```python
from build123d import *

# Parameters (mm, degrees)
SKETCH_R           = 9
PAD_DEPTH          = 6
POCKET_DEPTH       = 6
POLARPATTERN_COUNT = 16
SKETCH002_R        = 4
PAD001_DEPTH       = 6
SKETCH004_R        = 2
POCKET002_DEPTH    = 5
POCKET003_DEPTH    = 0.5
SKETCH003_R        = 1.25
POCKET004_DEPTH    = 15


with BuildPart() as part:
    # Sketch → Pad (new body)
    with BuildSketch(Plane.XY):
        Circle(SKETCH_R)
    extrude(amount=-PAD_DEPTH)

    # Sketch001 (on Face6 of Pad) → Pocket (cut)
    with BuildSketch(Plane.XY):
        Polygon((-0.5, 6.5), (0.5, 6.5), (0.75, 7.5), (1.25, 9), (-1.25, 9), (-0.75, 7.5), align=None)
    pocket = extrude(amount=-POCKET_DEPTH, mode=Mode.SUBTRACT)

    # PolarPattern: Pocket ×16 about axis
    polarpattern_axis = Axis((0, 0, 0), (0, 0, 1))
    for i in range(1, POLARPATTERN_COUNT):
        add(pocket.rotate(polarpattern_axis, i * 360 / POLARPATTERN_COUNT), mode=Mode.SUBTRACT)

    # Sketch002 → Pad001 (join)
    with BuildSketch(Plane.XY):
        Circle(SKETCH002_R)
    extrude(amount=PAD001_DEPTH)

    # Sketch004 → Pocket002 (cut)
    with BuildSketch(Plane.XZ):
        with Locations((0, 2.75)):
            Circle(SKETCH004_R)
    extrude(amount=POCKET002_DEPTH, mode=Mode.SUBTRACT)

    # Sketch004 → Pocket003 (cut)
    with BuildSketch(Plane.XZ):
        with Locations((0, 2.75)):
            Circle(SKETCH004_R)
    extrude(amount=-POCKET003_DEPTH, mode=Mode.SUBTRACT)

    # Sketch003 (on Face100 of Pad001) → Pocket004 (cut)
    with BuildSketch(Plane.XY.offset(6)):
        Circle(SKETCH003_R)
    extrude(amount=-POCKET004_DEPTH, mode=Mode.SUBTRACT)


solid = part.part
```
Read the model definition and answer for the solid it produces. Units are mm, in the model's axes. A direction names the side the tool comes from. Round coordinates to 2 decimals unless told otherwise and drop trailing zeros. Write each loop counter-clockwise with the first axis right and the second up, starting at its lowest first coordinate (ties: lowest second). Pieces come first, ordered by that corner, then holes. Notation, with made-up numbers: (16.5, 49.5) -> (24.5, 49.5) arc R16 ccw to (24.5, 59.5) -> close; hole circle Ø8 at (-12.5, 37). An arc over 180 degrees is marked (long way). Answer in a Markdown table with one row per item. Add a question column.
1) Which of the six approach directions +Z, -Z, +X, -X, +Y, -Y give full straight-line access (tool end or side, diameter ignored) to faces 4 (the face through (6.993, -0.623, -2.958)), 5 (the face through (6.7, 2.1, -3)), 6 (the face through (-6.993, 0.623, -2.958))?
2) Find section C-C, the plane z = 5. Determine the outline of the cut face in (x, y), and give its area (3 significant figures).
3) Determine the mould class of faces 1 (the face through (0.983, 8.198, -2.958)), 2 (the face through (5.1, -6.49, -2.96)), 3 (the face through (-6.23, -3.26, -2.96)) for opening direction X: pulls with the +X half, pulls with the -X half, needs draft (parallel to the pull), parting line crosses it, or undercut.
4) Consider line 1 (Y direction, x = 0, z = -0.25); line 2 (X direction, y = 4.5, z = -3.25); line 3 (X direction, y = 6.25, z = -2). Determine where each line is inside the solid, lowest interval first.
5) Find section B-B, the plane y = 0. Determine the outline of the cut face in (x, z), and give its area (3 significant figures).
6) Find section A-A, the plane x = 0. Determine the outline of the cut face in (y, z), and give its area (3 significant figures).
7) Find section D-D, the plane z = 2.75. Determine the outline of the cut face in (x, y), and give its area (3 significant figures).
8) Given P1, Ø1.5, axis at x = 2.5, z = -3, coming from the -Y side; P2, Ø8, axis at x = -6.5, y = -0.5, coming from the +Z side; P3, Ø5, axis at x = 0, z = 2.75, coming from the +Y side; P4, Ø0.5, axis at x = 0, z = -1.5, coming from the +Y side, each flat-ended and moving along its own axis, determine where each tip first touches the part or whether it passes through.
Findings below:
| question | item | result |
|---|---|---|
| 1 | face 4 | +Z, -Z, +X |
| 1 | face 5 | +Z, -Z |
| 1 | face 6 | +Z, -Z, -X |
| 2 | outline | circle Ø8 at (0, 0); hole circle Ø2.5 at (0, 0) |
| 2 | area | 45.4 mm² |
| 3 | face 1 | undercut |
| 3 | face 2 | pulls with the +X half |
| 3 | face 3 | pulls with the -X half |
| 4 | line 1 | -6.5 to -1.25, 1.25 to 6.5 |
| 4 | line 2 | -7.72 to -5.38, -4.69 to 4.69, 5.38 to 7.72 |
| 4 | line 3 | -4.98 to -3.27, -2.03 to 2.03, 3.27 to 4.98 |
| 5 | outline | (-6.5, -6) -> (-1.25, -6) -> (-1.25, 1.19) arc R2 cw to (-1.25, 4.31) -> (-1.25, 6) -> (-4, 6) -> (-4, 0) -> (-6.5, 0) -> close; (1.25, -6) -> (6.5, -6) -> (6.5, 0) -> (4, 0) -> (4, 6) -> (1.25, 6) -> (1.25, 4.31) arc R2 cw to (1.25, 1.19) -> close |
| 5 | area | 92.7 mm² |
| 6 | outline | (-6.5, -6) -> (-1.25, -6) -> (-1.25, 0.75) -> (-4, 0.75) -> (-4, 0) -> (-6.5, 0) -> close; (-4, 4.75) -> (-1.25, 4.75) -> (-1.25, 6) -> (-4, 6) -> close; (1.25, -6) -> (6.5, -6) -> (6.5, 0) -> (4, 0) -> (4, 6) -> (1.25, 6) -> close |
| 6 | area | 85.0 mm² |
| 7 | outline | (-2, -3.46) -> (-2, 0.5) -> (-1.15, 0.5) arc R1.25 cw to (1.15, 0.5) -> (2, 0.5) -> (2, -3.46) arc R4 ccw (long way) to start |
| 7 | area | 31.7 mm² |
| 8 | P1 | y = -8.83 |
| 8 | P2 | z = 6 |
| 8 | P3 | y = 4 |
| 8 | P4 | y = 6.5 |
